Work out the finished part from the listing and answer in its coordinate system (mm). Face numbers are marked on the shaded views. A direction names the side the tool comes from. Give positions to 0.01 mm unless a question says otherwise; leave off trailing zeros. Order: outer loops, then holes, each group sorted by start corner. A loop starts at its lowest first (then second) coordinate and runs counter-clockwise, first axis right, second up.
```python
from build123d import *

# Parameters (mm, degrees)
F0_W     = 8
F0_H     = 8
F0_R     = 1
F1_DEPTH = 2
F2_W     = 3
F2_H     = 8
F3_DEPTH = 2


with BuildPart() as f1:
    # F0 (on Top) → F1 (new body)
    with BuildSketch(Plane.XY):
        Rectangle(F0_W, F0_H)
        with Locations((-1.5, 0)):
            Circle(F0_R, mode=Mode.SUBTRACT)
    extrude(amount=F1_DEPTH)

    # F2 (on face) → F3 (join)
    with BuildSketch(Plane.XY.offset(2)):
        with Locations((2.5, 0)):
            Rectangle(F2_W, F2_H)
    extrude(amount=F3_DEPTH)


solid = f1.part
```
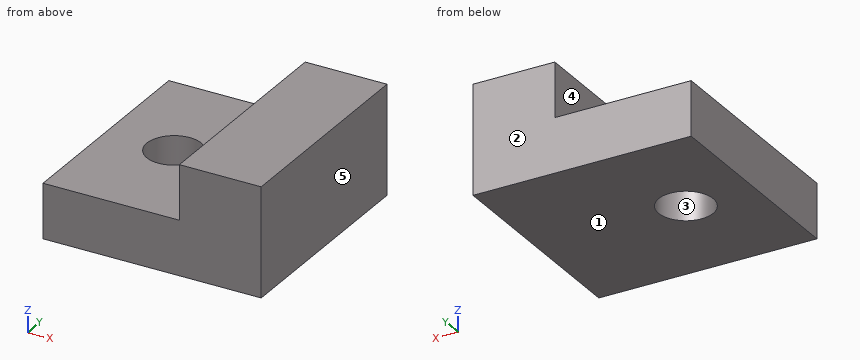
1. The part is cut by section A-A (x = -1.5). Write down the section's boundary in (y, z), then the cut area to 3 significant figures.
Findings below:
outline: (-4, 0) - (-1, 0) - (-1, 2) - (-4, 2) - close; (1, 0) - (4, 0) - (4, 2) - (1, 2) - close
area: 12.0 mm2
2. The part is cut by section B-B (y = 0). Write down the section's boundary in (x, z).
Findings below:
outline: (-4, 0) - (-2.5, 0) - (-2.5, 2) - (-4, 2) - close; (-0.5, 0) - (4, 0) - (4, 4) - (1, 4) - (1, 2) - (-0.5, 2) - close
3. Given P1, Ø2.5, axis at x = -1.5, y = 0, coming from the +Z side; P2, Ø1.6, axis at y = -2, z = 3, coming from the -X side, each flat-ended and moving along its own axis, determine where each tip first touches the part or whether it passes through.
Findings below:
P1: stops at z = 2
P2: stops at x = 1
4. Straight lines are drawn through the part: probe 1 along Y at (x, z) = (-1.5, 0.9); probe 2 along Z at (x, y) = (-1.5, 2.25); probe 3 along X at (y, z) = (1, 2.75). For each, find the intervals that lie inside material, in ascending order.
Findings below:
probe 1: y = -4 to -1, 1 to 4
probe 2: z = 0 to 2
probe 3: x = 1 to 4
5. The part is cut by section D-D (z = 3.5). Write down the section's boundary in (x, y), then the cut area to 3 significant figures.
Findings below:
outline: (1, -4) - (4, -4) - (4, 4) - (1, 4) - close
area: 24.0 mm2
6. The part is cut by section C-C (z = 1.8). Write down the section's boundary in (x, y), then the cut area to 3 significant figures.
Findings below:
outline: (-4, -4) - (4, -4) - (4, 4) - (-4, 4) - close; hole circle Ø2 at (-1.5, 0)
area: 60.9 mm2
7. Which of the six approach directions +Z, -Z, +X, -X, +Y, -Y give full straight-line access (tool end or side, diameter ignored) to the marked faces 4 and 5?
Findings below:
face 4: +Z, -X, +Y, -Y
face 5: +Z, -Z, +X, +Y, -Y
8. The mould has two halves that part along Y. Classify the marked faces 1, 2 and 3: pulls with the +Y half, pulls with the -Y half, needs draft (parallel to the pull), parting line crosses it, or undercut.
Findings below:
face 1: needs draft
face 2: pulls with the +Y half
face 3: undercut
